```python
from build123d import *

# Parameters (mm, degrees)
SKETCH_1_W               = 200
SKETCH_1_H               = 20
EXTRUDE_2_DEPTH          = 100
EXTRUDE_3_REACH          = 226.499
SKETCH_3_W               = 20
SKETCH_3_H               = 10
PATTERN_START            = -85
PATTERN_LINEAR_1_DEPTH   = 10
PATTERN_START_2          = -65
PATTERN_LINEAR_1_2_DEPTH = 10
PATTERN_START_3          = -45
PATTERN_LINEAR_1_3_DEPTH = 10
PATTERN_START_4          = -25
PATTERN_LINEAR_1_4_DEPTH = 10


# Read off the part's stored shape, not the designer's step: Линейный массив1
with BuildPart() as part:
    # Эскиз1 → Бобышка-Вытянуть2 (new body)
    with BuildSketch(Plane.XY):
        with Locations((100, 10)):
            Rectangle(SKETCH_1_W, SKETCH_1_H)
    extrude(amount=-EXTRUDE_2_DEPTH)

    # Бобышка-Вытянуть3: up to this plane
    extrude_3_end = Plane(origin=(-6.427876097, 17.660444431, 0), z_dir=(-0.34202014332566943, 0.9396926207859081, 0))
    # Эскиз3 → Бобышка-Вытянуть3 (add, up to the surface)
    with BuildSketch(Plane(origin=(0, 20, 0), x_dir=(1, 0, 0), z_dir=(0, 1, 0)), mode=Mode.PRIVATE) as extrude_3_sk1:
        with Locations((30, 20)):
            Rectangle(SKETCH_3_W, SKETCH_3_H)
    extrude_3_tool1 = split(extrude(extrude_3_sk1.sketch, amount=EXTRUDE_3_REACH, mode=Mode.PRIVATE), bisect_by=extrude_3_end, keep=Keep.BOTH, mode=Mode.PRIVATE)
    add(extrude_3_tool1.solids().sort_by_distance((30, 20, -20))[0])

    # Линейный массив1 outline → Линейный массив1 (add)
    with BuildSketch(Plane.XY.offset(PATTERN_START)):
        Polygon((170, 81.874939825), (170, 20), (190, 20), (190, 89.154344511), align=None)
        Polygon((120, 63.676428112), (120, 20), (140, 20), (140, 70.955832797), align=None)
        Polygon((70, 45.477916399), (70, 20), (90, 20), (90, 52.757321084), align=None)
        Polygon((20, 27.279404685), (20, 20), (40, 20), (40, 34.558809371), align=None)
    extrude(amount=PATTERN_LINEAR_1_DEPTH)

    # Pattern Linear 1 2 outline → Pattern Linear 1 2 (add)
    with BuildSketch(Plane.XY.offset(PATTERN_START_2)):
        Polygon((170, 81.874939825), (170, 20), (190, 20), (190, 89.154344511), align=None)
        Polygon((120, 63.676428112), (120, 20), (140, 20), (140, 70.955832797), align=None)
        Polygon((70, 45.477916399), (70, 20), (90, 20), (90, 52.757321084), align=None)
        Polygon((20, 27.279404685), (20, 20), (40, 20), (40, 34.558809371), align=None)
    extrude(amount=PATTERN_LINEAR_1_2_DEPTH)

    # Pattern Linear 1 3 outline → Pattern Linear 1 3 (add)
    with BuildSketch(Plane.XY.offset(PATTERN_START_3)):
        Polygon((170, 81.874939825), (170, 20), (190, 20), (190, 89.154344511), align=None)
        Polygon((120, 63.676428112), (120, 20), (140, 20), (140, 70.955832797), align=None)
        Polygon((70, 45.477916399), (70, 20), (90, 20), (90, 52.757321084), align=None)
        Polygon((20, 27.279404685), (20, 20), (40, 20), (40, 34.558809371), align=None)
    extrude(amount=PATTERN_LINEAR_1_3_DEPTH)

    # Pattern Linear 1 4 outline → Pattern Linear 1 4 (add)
    with BuildSketch(Plane.XY.offset(PATTERN_START_4)):
        Polygon((170, 81.874939825), (170, 20), (190, 20), (190, 89.154344511), align=None)
        Polygon((120, 63.676428112), (120, 20), (140, 20), (140, 70.955832797), align=None)
        Polygon((70, 45.477916399), (70, 20), (90, 20), (90, 52.757321084), align=None)
    extrude(amount=PATTERN_LINEAR_1_4_DEPTH)


solid = part.part
```
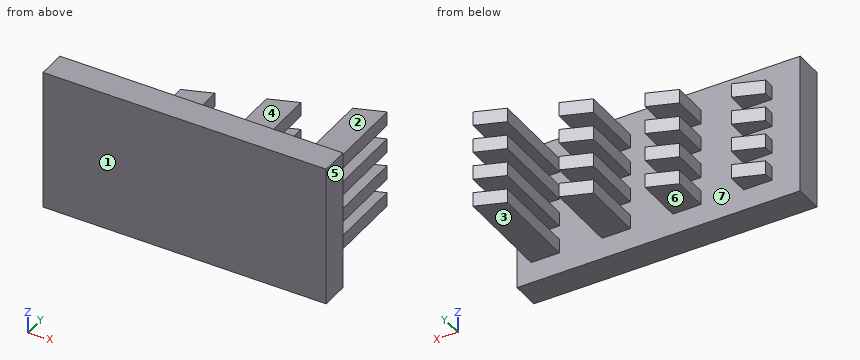
Design review of the part built by this model. Coordinates are the model's own, in mm. Face numbers are marked on the shaded views. A direction names the side the tool comes from. Give positions to 0.01 mm unless a question says otherwise; leave off trailing zeros. Write each loop counter-clockwise with the first axis right and the second up, starting at its lowest first coordinate (ties: lowest second). Pieces come first, ordered by that corner, then holes. Notation, with made-up numbers: (16.5, 28.25) - (75.5, 28.25) arc R16 cw to (75.5, 48.25) - close; hole circle Ø4 at (61, 26). An arc over 180 degrees is marked (long way). Return JSON: item names as keys, results as strings. Group by question number.
(1) We need section D-D, the plane y = 42.5. Give the number of separate pieces and of enclosed holes in the cut face, then the cut area to 3 significant figures.
(2) We need section B-B, the plane z = -22. Give the boundary of the cut face in (x, y).
(3) Machinability: for the marked faces 1, 2 and 3, which of the approach directions +Z, -Z, +X, -X, +Y, -Y give a long, thin tool a straight path to every point of the face, cutting with its end or side? Answer none if there is none.
(4) Insertion check: pin 1 (5 mm diameter, centred on x = 32.5, z = -51.5, fed in from +Y); pin 2 (11 mm diameter, centred on y = 26.5, z = -78.5, fed in from +X); pin 3 (6 mm diameter, centred on x = 180.5, y = 39, fed in from -Z). Each pin has a flat end and moves straight along its axis. Give the tip position at first contact, or say it passes through.
(5) Mouldability with a two-part tool opening along Z and no side actions: class the marked faces 4, 5, 6 and 7 as +Z half, -Z half, draft (parallel to the pull), parting line (faces both ways), or undercut.
(6) To check wall thickness, follow probe 1 along Z at (x, y) = (83.5, 39.5); probe 2 along X at (y, z) = (26, -44); probe 3 along Y at (x, z) = (39, -6). State the ranges of each line that lie inside material, in increasing order.
(7) We need section A-A, the plane y = 78.5. Give the boundary of the cut face in (x, z), then the cut area to 3 significant figures.
(8) We need section C-C, the plane x = 50. Give the boundary of the cut face in (y, z), then the cut area to 3 significant figures.
Reported:
{
 "1": {"separate pieces": "12", "enclosed holes": "0", "area": "2,400 mm2"},
 "2": {"outline": "(0, 0) - (200, 0) - (200, 20) - (190, 20) - (190, 89.15) - (170, 81.87) - (170, 20) - (140, 20) - (140, 70.96) - (120, 63.68) - (120, 20) - (90, 20) - (90, 52.76) - (70, 45.48) - (70, 20) - (40, 20) - (40, 34.56) - (20, 27.28) - (20, 20) - (0, 20) - close"},
 "3": {"face 1": "+Z, -Z, +X, -X, -Y", "face 2": "+Z, +X, -X, +Y", "face 3": "-Z, +X, -X, +Y"},
 "4": {"pin 1": "stops at y = 20", "pin 2": "stops at x = 190", "pin 3": "stops at z = -85"},
 "5": {"face 4": "+Z half", "face 5": "draft", "face 6": "-Z half", "face 7": "undercut"},
 "6": {"probe 1": "z = -85 to -75, -65 to -55, -45 to -35, -25 to -15", "probe 2": "x = 20 to 40, 70 to 90, 120 to 140, 170 to 190", "probe 3": "y = 0 to 20"},
 "7": {"outline": "(170, -85) - (190, -85) - (190, -75) - (170, -75) - close; (170, -65) - (190, -65) - (190, -55) - (170, -55) - close; (170, -45) - (190, -45) - (190, -35) - (170, -35) - close; (170, -25) - (190, -25) - (190, -15) - (170, -15) - close", "area": "800 mm2"},
 "8": {"outline": "(0, -100) - (20, -100) - (20, 0) - (0, 0) - close", "area": "2,000 mm2"}
}
